Can you work these out from the model? Positions are in its coordinate system, mm. Face numbers are marked on the shaded views. A direction names the side the tool comes from. Give positions to 0.01 mm unless a question says otherwise; leave off trailing zeros. Order: outer loops, then holes, each group sorted by start corner. A loop starts at its lowest first (then second) coordinate and runs counter-clockwise, first axis right, second up. Notation, with made-up numbers: (68.5, -39.5) - (96.5, -39.5) arc R15 ccw to (96.5, -31.5) - close; hole circle Ø2 at (84.5, 47). An arc over 180 degrees is marked (long way). One line per question, with ' | ' between items.
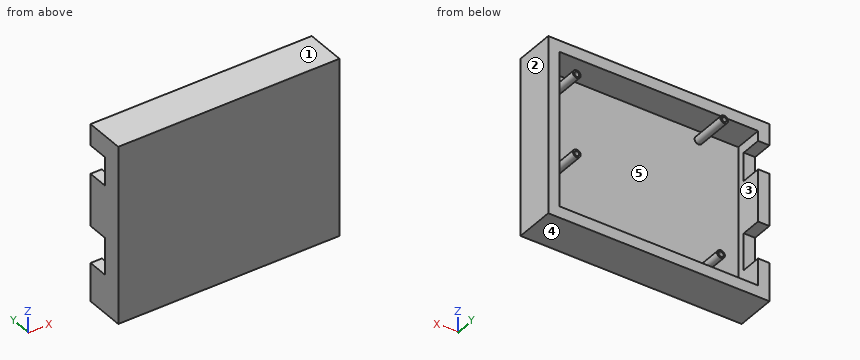
```python
from build123d import *

# Parameters (mm, degrees)
SKETCH1_W           = 77.9
SKETCH1_H           = 62.4
SKETCH1_W_2         = 69.9
SKETCH1_H_2         = 54.4
BOSS_EXTRUDE1_DEPTH = 10
SKETCH2_W           = 77.9
SKETCH2_H           = 62.4
BOSS_EXTRUDE2_DEPTH = 4
CUT_EXTRUDE1_REACH  = 99.872
SKETCH3_W           = 13
SKETCH3_H           = 7.25
CUT_EXTRUDE2_REACH  = 99.872
SKETCH4_W           = 10
SKETCH4_H           = 7.25
SKETCH5_R           = 1.36925
BOSS_EXTRUDE3_DEPTH = 17
SKETCH6_R           = 0.86925
CUT_EXTRUDE3_DEPTH  = 10


with BuildPart() as part:
    # Sketch1 → Boss-Extrude1 (new body)
    with BuildSketch(Plane(origin=(0, 0, 0), x_dir=(1, 0, 0), z_dir=(0, 1, 0))):
        with Locations((34.95, 27.2)):
            Rectangle(SKETCH1_W, SKETCH1_H)
        with Locations((34.95, 27.2)):
            Rectangle(SKETCH1_W_2, SKETCH1_H_2, mode=Mode.SUBTRACT)
    extrude(amount=BOSS_EXTRUDE1_DEPTH)

    # Sketch2 → Boss-Extrude2 (add)
    with BuildSketch(Plane(origin=(0, 0, 0), x_dir=(1, 0, 0), z_dir=(0, 1, 0))):
        with Locations((34.95, 27.2)):
            Rectangle(SKETCH2_W, SKETCH2_H)
    extrude(amount=-BOSS_EXTRUDE2_DEPTH)

    # Sketch3 → Cut-Extrude1 (cut, up to next)
    with BuildSketch(Plane.ZY.offset(4), mode=Mode.PRIVATE) as cut_extrude1_sk1:
        with Locations((-38.4, 6.375)):
            Rectangle(SKETCH3_W, SKETCH3_H)
    cut_extrude1_tool1 = extrude(cut_extrude1_sk1.sketch, amount=-CUT_EXTRUDE1_REACH, mode=Mode.PRIVATE) & part.part
    add(cut_extrude1_tool1.solids().sort_by_distance((-4, 6.375, -38.4))[0], mode=Mode.SUBTRACT)

    # Sketch4 → Cut-Extrude2 (cut, up to next)
    with BuildSketch(Plane.ZY.offset(4), mode=Mode.PRIVATE) as cut_extrude2_sk1:
        with Locations((-8.5, 6.375)):
            Rectangle(SKETCH4_W, SKETCH4_H)
    cut_extrude2_tool1 = extrude(cut_extrude2_sk1.sketch, amount=-CUT_EXTRUDE2_REACH, mode=Mode.PRIVATE) & part.part
    add(cut_extrude2_tool1.solids().sort_by_distance((-4, 6.375, -8.5))[0], mode=Mode.SUBTRACT)

    # Sketch5 → Boss-Extrude3 (add)
    with BuildSketch(Plane(origin=(0, -4, 0), x_dir=(-1, 0, 0), z_dir=(0, -1, 0))):
        with Locations(Location((-65.94475, 7.99125, 0), (0, 0, 90))):
            Circle(SKETCH5_R)
        with Locations(Location((-15.15745, 51.15855, 0), (0, 0, 90))):
            Circle(SKETCH5_R)
        with Locations(Location((-65.94475, 35.91855, 0), (0, 0, 90))):
            Circle(SKETCH5_R)
        with Locations(Location((-14.01445, 3.24145, 0), (0, 0, 90))):
            Circle(SKETCH5_R)
    extrude(amount=-BOSS_EXTRUDE3_DEPTH)

    # Sketch6 → Cut-Extrude3 (cut)
    with BuildSketch(Plane(origin=(0, 13, 0), x_dir=(1, 0, 0), z_dir=(0, 1, 0))):
        with Locations(Location((65.94475, 35.91855, 0), (0, 0, 270))):
            Circle(SKETCH6_R)
        with Locations(Location((65.94475, 7.99125, 0), (0, 0, 270))):
            Circle(SKETCH6_R)
        with Locations(Location((14.01445, 3.24145, 0), (0, 0, 270))):
            Circle(SKETCH6_R)
        with Locations(Location((15.15745, 51.15855, 0), (0, 0, 270))):
            Circle(SKETCH6_R)
    extrude(amount=-CUT_EXTRUDE3_DEPTH, mode=Mode.SUBTRACT)


solid = part.part
```
(1) Imagine slicing it at C-C (z = -28). List the corners of the cut face in (x, y) for me, and give its area (3 significant figures).
Answer below:
outline: (-4, -4) - (73.9, -4) - (73.9, 10) - (69.9, 10) - (69.9, 0) - (0, 0) - (0, 10) - (-4, 10) - close | area: 392 mm^2
(2) Imagine slicing it at B-B (y = 11.5). List the corners of the cut face in (x, z) for me.
Answer below:
outline: circle Ø2.74 at (14.01, -3.24); circle Ø2.74 at (15.16, -51.16); circle Ø2.74 at (65.94, -35.92); circle Ø2.74 at (65.94, -7.99); hole circle Ø1.74 at (14.01, -3.24); hole circle Ø1.74 at (15.16, -51.16); hole circle Ø1.74 at (65.94, -35.92); hole circle Ø1.74 at (65.94, -7.99)
(3) Imagine slicing it at A-A (y = 5). Count the separate pieces of the cut face and the enclosed holes in it, and give its area (3 significant figures).
Answer below:
separate pieces: 6 | enclosed holes: 4 | area: 980 mm^2
(4) If I drill on line 1 (X direction, y = 6.5, z = -20); line 2 (Z direction, x = 53, y = 7.5); line 3 (X direction, y = 12, z = -36), over which ranges is the centre line in solid material (lowest first)?
Answer below:
line 1: -4 to 0, 69.9 to 73.9 | line 2: -58.4 to -54.4, 0 to 4 | line 3: 64.58 to 65.08, 66.81 to 67.31
(5) Imagine slicing it at D-D (x = 30). List the corners of the cut face in (y, z) for me.
Answer below:
outline: (-4, -58.4) - (10, -58.4) - (10, -54.4) - (0, -54.4) - (0, 0) - (10, 0) - (10, 4) - (-4, 4) - close
(6) On a 3-axis mill with a long thin cutter (end or side, diameter ignored), from which of +Z, -Z, +X, -X, +Y, -Y can I reach the whole of each face in a straight line? I mean the marked faces 4 and 5. Say none if no direction works.
Answer below:
face 4: -Z, +X, -X, +Y, -Y | face 5: +Y
(7) If we mould it in two halves opening along X, with no side actions, what happens to the marked faces 1, 2 and 3? For each: released by +X, released by -X, zero draft, split by the parting line, or undercut.
Answer below:
face 1: zero draft | face 2: released by +X | face 3: undercut
(8) Will these pins go through, and if not, where does the flat tip stop? pin 1 (1 mm diameter, centred on x = 65.94, z = -35.92, fed in from +Y); pin 2 (2 mm diameter, centred on x = -1.5, z = -26.5, fed in from +Y); pin 3 (1.9 mm diameter, centred on x = 14, z = -3, fed in from +Y); pin 4 (1 mm diameter, centred on x = 49.5, z = -8, fed in from +Y).
Answer below:
pin 1: y = 3 | pin 2: y = 10 | pin 3: y = 13 | pin 4: y = 0
